Geometry: final body of the model. Coordinates: model frame, mm. A direction names the side the tool comes from. Coordinates: 2 decimals unless noted, no trailing zeros. Order: outer loops, then holes, each group sorted by start corner. A loop starts at its lowest first (then second) coordinate and runs counter-clockwise, first axis right, second up. Notation, with made-up numbers: M -32,14 L -21,14 A33 cw -21,45 Z; hole C -17.5,26 d1. An arc over 180 degrees is marked long. Use CSV: the item, a comma, the result in double quotes. Start each with the question number.
1. Section query B-B on z = -1.25. State how many separate pieces and enclosed holes the cut face has, and give its area (3 significant figures).
2. Material intervals for line 1 (X direction, y = -23, z = -3.5); line 2 (X direction, y = 13, z = -5); line 3 (X direction, y = -8.5, z = -5), sorted ascending.
3. First-contact query: P1, Ø3.5, axis at x = -63.41, y = -19.61, coming from the -Z side; P2, Ø1.5, axis at x = 46, z = -5, coming from the -Y side; P3, Ø5.5, axis at x = -60.33, y = -55.73, coming from the +Z side. Flat tips, straight axial feed; report the tip coordinate or a pass-through.
4. Set-up query: faces 1 (the cylindrical face through (-59.236, -22.983, -1.343)), 2 (the flat face through (-63.65, 27.49, -4.51)), 3 (the cylindrical face through (42.04, 67.62, -3.22)). Return all of +Z, -Z, +X, -X, +Y, -Y with unobstructed straight access to the full face (end or side cutting, diameter ignored); none if empty.
5. Section query A-A on y = 10. Return the cut outline in (x, z) (3 decimals).
Autodesk Inventor part; units mm, degrees
ref_plane "YZ Plane" through (0, 0, 0) normal (1, 0, 0) x (0, 1, 0)
ref_plane "XZ Plane" through (0, 0, 0) normal (0, 1, 0) x (-1, 0, 0)
ref_plane "XY Plane" through (0, 0, 0) normal (0, 0, 1) x (1, 0, 0)
sketch "Sketch1" plane through (0, 0, 0) normal (0, 0, 1) x (1, 0, 0)
  circle A0 centre (49.935, 18.1273) radius 2.15
  circle A1 centre (22.1322, -42.1716) radius 2.15
  circle A2 centre (-10.364, 45.9302) radius 2.15
  circle A3 centre (-21.2973, -38.0061) radius 2 construction
  circle A4 centre (-43.3867, -61.1591) radius 2 construction
  circle A5 centre (-66.5396, -39.0697) radius 2 construction
  circle A6 centre (-44.4503, -15.9167) radius 2 construction
  circle A7 centre (-21.2973, -38.0061) radius 2.15
  circle A8 centre (-43.3867, -61.1591) radius 2.15
  circle A9 centre (-66.5396, -39.0697) radius 2.15
  circle A10 centre (-44.4503, -15.9167) radius 2.15
  line L0 (72.7593, -34.944) -> (-63.7175, -74.4952)
  circle A11 centre (22.1322, -42.1716) radius 7.15 construction
  circle A12 centre (-43.3867, -61.1591) radius 7.15 construction
  circle A13 centre (49.935, 18.1273) radius 7.15 construction
  circle A14 centre (-10.364, 45.9302) radius 7.15 construction
  line L1 (72.7593, -34.944) -> (42.7074, 68.7545)
  line L2 (61.4193, 4.1865) -> (59.0868, 12.2348)
  line L3 (42.7074, 68.7545) -> (-93.7695, 29.2033)
  circle A15 centre (-66.5396, -39.0697) radius 7.15 construction
  line L4 (-63.7175, -74.4952) -> (-93.7695, 29.2033)
  arc A16 (26.2989, -37.6054) -> (49.1681, 11.9935) centre (5.8841, 1.8793) ccw construction
  circle A17 centre (5.8841, 1.8793) radius 44.45
  arc A18 (-43.4778, -57.2827) -> (-49.2361, -56.518) centre (-43.9185, -38.5379) ccw construction
  circle A19 centre (-43.9185, -38.5379) radius 18.75
  circle A20 centre (-41.0626, 2.5767) radius 2.15
  point P0 (0, 0)
  dimension "d4" = 4.3
  dimension "d5" = 4.3
  dimension "d6" = 4.3
  dimension "d7" = 4.3
  dimension "d8" = 5
  dimension "d10" = 0
  dimension "d11" = 5
  dimension "d12" = 5
  dimension "d13" = 0
  dimension "d14" = 5
  dimension "d15" = 5
extrude "Extrusion1" add sketch "Sketch1" against normal blind 6.35
sketch "Sketch3" plane through (0, 0, 0) normal (0, 0, 1) x (1, 0, 0)
  line L0 (-61.3029, 24.5377) -> (-55.2691, 23.1116)
  line L1 (-55.2691, 23.1116) -> (-55.1667, 23.5451)
  arc A0 (-55.1667, 23.5451) -> (-61.2004, 24.9712) centre (-59.9421, 16.8177) ccw
  line L2 (-61.2004, 24.9712) -> (-61.3029, 24.5377)
  arc A1 (-66.2644, 27.4572) -> (-68.0692, 26.3425) centre (-66.6094, 25.9974) ccw
  line L3 (-66.2644, 27.4572) -> (-49.5256, 23.501)
  arc A2 (-48.4108, 21.6962) -> (-49.5256, 23.501) centre (-49.8706, 22.0412) ccw
  line L4 (-48.4108, 21.6962) -> (-57.1054, -15.0903)
  arc A3 (-58.9102, -16.2051) -> (-57.1054, -15.0903) centre (-58.5652, -14.7453) ccw
  line L5 (-58.9102, -16.2051) -> (-75.649, -12.2488)
  arc A4 (-76.7638, -10.444) -> (-75.649, -12.2488) centre (-75.304, -10.789) ccw
  line L6 (-76.7638, -10.444) -> (-68.0692, 26.3425)
  line L7 (-48.0658, 23.1559) -> (-67.7242, 27.8022)
  line L8 (-67.7242, 27.8022) -> (-66.1486, 34.4686)
  line L9 (-66.1486, 34.4686) -> (-46.4902, 29.8223)
  line L10 (-46.4902, 29.8223) -> (-48.0658, 23.1559)
  line L11 (-48.0658, 23.1559) -> (-48.4722, 21.4367)
  line L12 (-67.7242, 27.8022) -> (-68.3933, 24.9712)
  line L13 (-52.7581, 3.3029) -> (-72.4165, 7.9492) construction
  line L14 (-75.649, -12.2488) -> (-58.9102, -16.2051)
  line L15 (-57.4504, -16.5501) -> (-77.1088, -11.9038)
  line L16 (-77.1088, -11.9038) -> (-78.6844, -18.5701)
  line L17 (-78.6844, -18.5701) -> (-59.026, -23.2164)
  line L18 (-59.026, -23.2164) -> (-57.4504, -16.5501)
  line L19 (-57.4504, -16.5501) -> (-57.1054, -15.0903)
  line L20 (-77.1088, -11.9038) -> (-76.7638, -10.444)
  line L21 (-59.026, -23.2164) -> (-78.6844, -18.5701)
  line L22 (-78.6844, -18.5701) -> (-66.1486, 34.4686)
  line L23 (-66.1486, 34.4686) -> (-46.4902, 29.8223)
  line L24 (-46.4902, 29.8223) -> (-59.026, -23.2164)
  line L25 (-56.9137, -19.8007) -> (-46.1306, 25.8223)
  line L26 (-49.9059, 31.9346) -> (-62.1486, 34.8282)
  line L27 (-68.2609, 31.0529) -> (-79.044, -14.5701)
  line L28 (-75.2687, -20.6824) -> (-63.026, -23.576)
  arc A5 (-46.1306, 25.8223) -> (-49.9059, 31.9346) centre (-51.0744, 26.9908) ccw
  arc A6 (-62.1486, 34.8282) -> (-68.2609, 31.0529) centre (-63.3171, 29.8844) ccw
  arc A7 (-63.026, -23.576) -> (-56.9137, -19.8007) centre (-61.8575, -18.6322) ccw
  arc A8 (-79.044, -14.5701) -> (-75.2687, -20.6824) centre (-74.1002, -15.7386) ccw
  point P0 (0, 0)
  point P1 (-58.0822, -24.7445)
  point P2 (-44.9621, 30.7661)
  point P3 (-67.0924, 35.9966)
  point P4 (-80.2125, -19.5139)
  point P5 (-66.2644, 27.4572)
  point P6 (-46.5937, 29.3844)
  point P7 (-46.928, 29.9257)
  point P8 (-65.7107, 34.3651)
  point P9 (-66.2521, 34.0307)
  point P10 (-78.5809, -18.1323)
  point P11 (-78.2466, -18.6736)
  point P12 (-59.4639, -23.1129)
  point P13 (-58.9226, -22.7786)
  dimension "d18" = 6.85
  dimension "d19" = 0
  dimension "d20" = 0
  dimension "d23" = 1.27
  dimension "d24" = 1.27
  dimension "d25" = 9.62
  dimension "d26" = 21.47
  dimension "d27" = 8.12
  dimension "d28" = 5.08
extrude "Extrusion2" cut sketch "Sketch3" against normal blind 2.725 contours L2 A0 L1 L0 | L3 A2 L4 A3 L5 A4 L6 A1 | L7 L8 A6 L9 A5 L10 L3 | A1 L12 L7 | L6 L20 L16 A8 L27 A6 L8 L12 | L7 L11 A2 | L11 L10 A5 L25 A7 L18 L19 L4 | A4 L15 L20 | A6 L26 A5 L9 | L5 L15 L18 A7 L17 A8 L16 | L19 L15 A3 | L17 A7 L28 A8
sketch "Sketch4" plane through (0, 0, -2.725) normal (0, 0, 1) x (1, 0, 0)
  line L0 (-61.3029, 24.5377) -> (-55.2691, 23.1116) construction
  line L1 (-55.2691, 23.1116) -> (-55.1667, 23.5451) construction
  arc A0 (-55.1667, 23.5451) -> (-61.2004, 24.9712) centre (-59.9421, 16.8177) ccw construction
  line L2 (-61.2004, 24.9712) -> (-61.3029, 24.5377) construction
  line L3 (-66.2644, 27.4572) -> (-49.5256, 23.501)
  arc A1 (-48.4108, 21.6962) -> (-49.5256, 23.501) centre (-49.8706, 22.0412) ccw construction
  line L4 (-46.9502, 27.8759) -> (-48.4108, 21.6962) construction
  arc A2 (-46.9502, 27.8759) -> (-48.4366, 30.2823) centre (-48.8966, 28.3359) ccw construction
  line L5 (-49.9937, 30.6503) -> (-48.4366, 30.2823) construction
  line L6 (-50.1677, 29.9142) -> (-49.9937, 30.6503) construction
  arc A3 (-53.0872, 30.6042) -> (-50.1677, 29.9142) centre (-52.0285, 28.5624) ccw construction
  line L7 (-52.9132, 31.3404) -> (-53.0872, 30.6042) construction
  line L8 (-59.7255, 32.9505) -> (-52.9132, 31.3404) construction
  line L9 (-59.8995, 32.2143) -> (-59.7255, 32.9505) construction
  arc A4 (-62.8191, 32.9044) -> (-59.8995, 32.2143) centre (-61.7604, 30.8625) ccw construction
  line L10 (-62.6451, 33.6405) -> (-62.8191, 32.9044) construction
  line L11 (-64.2022, 34.0085) -> (-62.6451, 33.6405) construction
  arc A5 (-64.2022, 34.0085) -> (-66.6086, 32.5222) centre (-64.6622, 32.0622) ccw construction
  line L12 (-68.0692, 26.3425) -> (-66.6086, 32.5222) construction
  arc A6 (-66.2644, 27.4572) -> (-68.0692, 26.3425) centre (-66.6094, 25.9974) ccw construction
  line L13 (-48.4108, 21.6962) -> (-57.1054, -15.0903) construction
  arc A7 (-60.9724, -22.7564) -> (-58.566, -21.2701) centre (-60.5124, -20.81) ccw construction
  line L14 (-60.9724, -22.7564) -> (-62.5295, -22.3884) construction
  line L15 (-62.5295, -22.3884) -> (-62.3555, -21.6522) construction
  arc A8 (-62.3555, -21.6522) -> (-65.2751, -20.9622) centre (-63.4143, -19.6104) ccw construction
  line L16 (-65.2751, -20.9622) -> (-65.4491, -21.6983) construction
  line L17 (-65.4491, -21.6983) -> (-72.2614, -20.0882) construction
  line L18 (-72.2614, -20.0882) -> (-72.0874, -19.3521) construction
  arc A9 (-72.0874, -19.3521) -> (-75.007, -18.662) centre (-73.1461, -17.3102) ccw construction
  line L19 (-75.007, -18.662) -> (-75.181, -19.3982) construction
  line L20 (-75.181, -19.3982) -> (-76.738, -19.0301) construction
  arc A10 (-78.2244, -16.6237) -> (-76.738, -19.0301) centre (-76.278, -17.0838) ccw construction
  line L21 (-78.2244, -16.6237) -> (-76.7638, -10.444) construction
  line L22 (-76.7638, -10.444) -> (-68.0692, 26.3425) construction
  arc A11 (-58.9102, -16.2051) -> (-57.1054, -15.0903) centre (-58.5652, -14.7453) ccw construction
  line L23 (-58.9102, -16.2051) -> (-75.649, -12.2488) construction
  arc A12 (-76.7638, -10.444) -> (-75.649, -12.2488) centre (-75.304, -10.789) ccw construction
  circle A13 centre (-52.0285, 28.5624) radius 2.15
  circle A14 centre (-61.7604, 30.8625) radius 2.15
  circle A15 centre (-63.4143, -19.6104) radius 2.15
  circle A16 centre (-73.1461, -17.3102) radius 2.15
  line L24 (-54.4118, 21.5218) -> (-54.1473, 22.641) construction
  line L25 (-62.5167, 24.6191) -> (-62.7812, 23.4999) construction
  circle A17 centre (-52.0285, 28.5624) radius 3 construction
  circle A18 centre (-61.7604, 30.8625) radius 3 construction
  line L26 (-55.9486, 25.0191) -> (-59.8414, 25.9391) construction
  line L27 (-59.8414, 25.9391) -> (-58.5579, 31.3695)
  line L28 (-58.5579, 31.3695) -> (-54.6651, 30.4494)
  line L29 (-54.6651, 30.4494) -> (-55.9486, 25.0191)
  line L30 (-56.4874, -15.2364) -> (-47.7929, 21.5501)
  arc A19 (-47.7929, 21.5501) -> (-49.3795, 24.1189) centre (-49.8706, 22.0412) ccw
  line L31 (-49.3795, 24.1189) -> (-66.1183, 28.0752)
  arc A20 (-66.1183, 28.0752) -> (-68.6872, 26.4885) centre (-66.6094, 25.9974) ccw
  line L32 (-68.6872, 26.4885) -> (-77.3818, -10.2979)
  line L33 (-77.3818, -10.2979) -> (-78.8424, -16.4777)
  arc A21 (-78.8424, -16.4777) -> (-76.8841, -19.6481) centre (-76.278, -17.0838) ccw
  line L34 (-76.8841, -19.6481) -> (-74.709, -20.1622)
  line L35 (-74.709, -20.1622) -> (-74.3152, -18.4958)
  arc A22 (-72.6316, -18.8937) -> (-74.3152, -18.4958) centre (-73.1461, -17.3102) ccw
  line L36 (-72.6316, -18.8937) -> (-73.0254, -20.5601)
  line L37 (-73.0254, -20.5601) -> (-64.9772, -22.4624)
  line L38 (-64.9772, -22.4624) -> (-64.5833, -20.7959)
  arc A23 (-62.8997, -21.1939) -> (-64.5833, -20.7959) centre (-63.4143, -19.6104) ccw
  line L39 (-62.8997, -21.1939) -> (-63.2936, -22.8603)
  line L40 (-63.2936, -22.8603) -> (-61.1185, -23.3744)
  arc A24 (-61.1185, -23.3744) -> (-57.948, -21.4161) centre (-60.5124, -20.81) ccw
  line L41 (-75.7951, -12.8668) -> (-59.0563, -16.823)
  arc A25 (-59.0563, -16.823) -> (-56.4874, -15.2364) centre (-58.5652, -14.7453) ccw
  line L42 (-56.4874, -15.2364) -> (-47.7929, 21.5501)
  line L43 (-47.7929, 21.5501) -> (-46.3323, 27.7298)
  arc A26 (-46.3323, 27.7298) -> (-48.2905, 30.9003) centre (-48.8966, 28.3359) ccw
  line L44 (-48.2905, 30.9003) -> (-50.4656, 31.4144)
  line L45 (-50.4656, 31.4144) -> (-50.8594, 29.7479)
  arc A27 (-52.5431, 30.1459) -> (-50.8594, 29.7479) centre (-52.0285, 28.5624) ccw
  line L46 (-52.5431, 30.1459) -> (-52.1492, 31.8123)
  line L47 (-52.1492, 31.8123) -> (-60.1975, 33.7145)
  line L48 (-60.1975, 33.7145) -> (-60.5913, 32.0481)
  arc A28 (-62.2749, 32.446) -> (-60.5913, 32.0481) centre (-61.7604, 30.8625) ccw
  line L49 (-62.2749, 32.446) -> (-61.8811, 34.1124)
  line L50 (-61.8811, 34.1124) -> (-64.0561, 34.6265)
  arc A29 (-64.0561, 34.6265) -> (-67.2266, 32.6683) centre (-64.6622, 32.0622) ccw
  line L51 (-67.2266, 32.6683) -> (-68.6872, 26.4885)
  line L52 (-68.6872, 26.4885) -> (-77.3818, -10.2979)
  arc A30 (-77.3818, -10.2979) -> (-75.7951, -12.8668) centre (-75.304, -10.789) ccw
  point P0 (0, 0)
  point P1 (-56.3194, 32.1454)
  point P2 (-55.8026, 25.637)
  point P3 (-59.6953, 26.5571)
  point P4 (-74.4407, -19.0268)
  point P5 (-72.7571, -19.4247)
  point P6 (-64.7088, -21.327)
  point P7 (-63.0252, -21.7249)
  point P8 (-77.3818, -10.2979)
  dimension "d29" = 4.3
  dimension "d30" = 4.3
  dimension "d31" = 4.3
  dimension "d32" = 4.3
  dimension "d33" = 6
  dimension "d34" = 6
  dimension "d35" = 1.27
  dimension "d36" = 0
  dimension "d39" = 0.635
  dimension "d41" = 0.635
extrude "Extrusion3" cut sketch "Sketch4" against normal through all contours L27 L31 L29 L3 | L3 L29 L31 A19 L30 A25 L41 A30 L32 A20 L27 | L27 L28 L29 L31 | A15 L39 A23 L38 | L38 A23 L39 A15 | A16 L36 A22 L35 | L35 A22 L36 A16 | L49 A28 L48 A14 | A14 L48 A28 L49 | L45 A27 L46 A13 | A13 L46 A27 L45
fillet "Fillet1" radius 1.5875 4 edges at (-55.8026, 25.637, -4.5375) (-54.6651, 30.4494, -4.5375) (-58.5579, 31.3695, -4.5375) (-59.6953, 26.5571, -4.5375)
fillet "Fillet2" radius 3.175 1 edges at (42.7074, 68.7545, -3.175)
sketch "Sketch5" plane through (0, 0, 0) normal (0, 0, 1) x (1, 0, 0)
  circle A0 centre (57.0512, -21.713) radius 2.15
  circle A1 centre (34.6484, 55.5908) radius 2.15
  circle A2 centre (-82.7345, 21.5731) radius 2.15
  circle A3 centre (-60.3318, -55.7307) radius 2.15
  circle A4 centre (57.0512, -21.713) radius 3.05
  circle A5 centre (34.6484, 55.5908) radius 3.05
  circle A6 centre (-82.7345, 21.5731) radius 3.05
  circle A7 centre (-60.3318, -55.7307) radius 3.05
  point P0 (0, 0)
  dimension "d43" = 6.1
  dimension "d44" = 6.1
  dimension "d45" = 6.1
  dimension "d46" = 6.1
extrude "Extrusion4" cut sketch "Sketch5" against normal blind 0.15
sketch "Sketch6" plane through (-60.3318, -55.7307, 0) normal (0, 0, 1) x (1, 0, 0)
  circle A0 centre (-22.4027, 77.3038) radius 2.15
  circle A1 centre (94.9802, 111.3215) radius 2.15
  circle A2 centre (117.383, 34.0177) radius 2.15
  circle A3 centre (0, 0) radius 2.15
  point P0 (60.3318, 55.7307)
extrude "Extrusion5" cut sketch "Sketch6" against normal through all
properties part number "Lower_Plate"
Results list:
1,separate pieces,"1"
1,enclosed holes,"15"
1,area,"6,580 mm²"
2,line 1,"x = -78.64 to -54.41, -33.42 to -30.95, 42.72 to 55.33, 58.77 to 69.3"
2,line 2,"x = -89.07 to -71.88, -49.81 to -37.15, 48.92 to 58.87"
2,line 3,"x = -82.84 to -76.96, -54.9 to -37.34, 49.11 to 65.1"
3,P1,"passes through"
3,P2,"stops at y = -42.92"
3,P3,"stops at z = -0.15"
4,face 1,"+Z"
4,face 2,"+Z, -Z"
4,face 3,"+Z, -Z, +Y"
5,outline,"M -88.204,-6.35 L -72.584,-6.35 L -72.584,-2.725 L -73.237,-2.725 L -73.237,0 L -88.204,0 Z; M -50.523,-6.35 L -37.818,-6.35 L -37.818,0 L -49.87,0 L -49.87,-2.725 L -50.523,-2.725 Z; M 49.586,-6.35 L 59.734,-6.35 L 59.734,0 L 49.586,0 Z"
